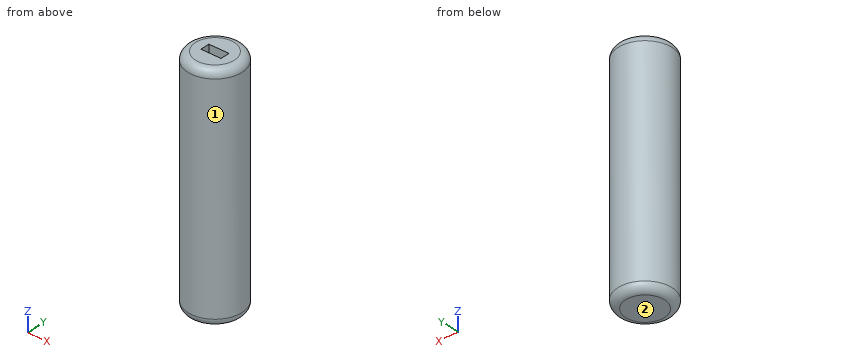
```python
from build123d import *

# Parameters (mm, degrees)
F0_R     = 17.5
F1_DEPTH = 150
F2_W     = 13
F2_H     = 6
F3_DEPTH = 87
F4_R     = 1.960614
F5_DEPTH = 20
F6_R     = 5


with BuildPart() as f1:
    # F0 (on Top) → F1 (new body)
    with BuildSketch(Plane.XY):
        Circle(F0_R)
    extrude(amount=F1_DEPTH)

    # F2 (on face) → F3 (cut)
    with BuildSketch(Plane.XY.offset(150)):
        Rectangle(F2_W, F2_H)
    extrude(amount=-F3_DEPTH, mode=Mode.SUBTRACT)

    # F4 (on face) → F5 (cut)
    with BuildSketch(Plane.XY.offset(63)):
        Circle(F4_R)
    extrude(amount=-F5_DEPTH, mode=Mode.SUBTRACT)

    # F6
    f6_edges = [f1.edges().sort_by_distance(p)[0] for p in [
        (-17.5, 0, 150),
        (-17.5, 0, 0),
    ]]
    fillet(f6_edges, radius=F6_R)


solid = f1.part
```
Check sheet for the modelled part. Datum: model origin and axes. Units: mm. Face numbers are marked on the shaded views. Round coordinates to 2 decimals unless told otherwise and drop trailing zeros. Order: outer loops, then holes, each group sorted by start corner. A loop starts at its lowest first (then second) coordinate and runs counter-clockwise, first axis right, second up.
1) Section check D-D (z = 54.5). Record the boundary of the cut face in (x, y).
2) Go/stop test with flat-tipped pins: pin 1 Ø3.5 at (x, y) = (0, 0) entering from -Z; pin 2 Ø1.5 at (x, z) = (-2, 125.5) entering from +Y; pin 3 Ø12 at (y, z) = (-8.5, 130.5) entering from -X; pin 4 Ø8 at (y, z) = (-12.5, 20.5) entering from +X. Record where each tip stops, or that it passes through.
3) Section check B-B (y = 0). Record the boundary of the cut face in (x, z).
4) Section check A-A (x = 0). Record the boundary of the cut face in (y, z), and give its area (3 significant figures).
5) Mould release check, pull along X, two halves, no side actions. Record for the marked faces 1 and 2: +X half, -X half, draft (parallel to the pull), parting line (faces both ways), or undercut.
6) Scan lines: line 1 (Y direction, x = 0, z = 58); line 2 (Z direction, x = 3.5, y = 1); line 3 (Z direction, x = -12, y = 4). Record each from-to range of solid material in increasing order.
7) Section check C-C (z = 73). Record the boundary of the cut face in (x, y), and give its area (3 significant figures).
Result:
1. outline: circle Ø35 at (0, 0); hole circle Ø3.92 at (0, 0)
2. pin 1: stops at z = 0
2. pin 2: stops at y = 17.46
2. pin 3: stops at x = -17.32
2. pin 4: stops at x = 15.3
3. outline: (-17.5, 5) arc R5 ccw to (-12.5, 0) - (12.5, 0) arc R5 ccw to (17.5, 5) - (17.5, 145) arc R5 ccw to (12.5, 150) - (6.5, 150) - (6.5, 63) - (1.96, 63) - (1.96, 43) - (-1.96, 43) - (-1.96, 63) - (-6.5, 63) - (-6.5, 150) - (-12.5, 150) arc R5 ccw to (-17.5, 145) - close
4. outline: (-17.5, 5) arc R5 ccw to (-12.5, 0) - (12.5, 0) arc R5 ccw to (17.5, 5) - (17.5, 145) arc R5 ccw to (12.5, 150) - (3, 150) - (3, 63) - (1.96, 63) - (1.96, 43) - (-1.96, 43) - (-1.96, 63) - (-3, 63) - (-3, 150) - (-12.5, 150) arc R5 ccw to (-17.5, 145) - close
4. area: 4,630 mm2
5. face 1: parting line
5. face 2: draft
6. line 1: y = -17.5 to -1.96, 1.96 to 17.5
6. line 2: z = 0 to 63
6. line 3: z = 0 to 150
7. outline: circle Ø35 at (0, 0); hole (-6.5, -3) - (6.5, -3) - (6.5, 3) - (-6.5, 3) - close
7. area: 884 mm2
